Model file for the job. Use its own axes, mm. Face numbers are marked on the shaded views. A direction names the side the tool comes from. Round coordinates to 2 decimals unless told otherwise and drop trailing zeros. Loops run counter-clockwise (first coordinate to the right, second up) from the corner with the lowest first, then second, coordinate; pieces in that order, holes last. Notation, with made-up numbers: (75.5, 5) - (122.5, 5) arc R23 cw to (122.5, 13) - close; hole circle Ø7 at (71, 84). An arc over 180 degrees is marked (long way). Answer as a JSON object with one key per item and string values.
from build123d import *

# Parameters (mm, degrees)
F2_W = 40.0049984455
F2_H = 8.5304779932


with BuildPart() as f1:
    # F0 (on Front) → F1 (revolve)
    with BuildSketch(Plane.XZ):
        with BuildLine():
            Line((-17.918098104, 0), (0, 0))
            Line((0, 0), (0, 10.5895595625))
            Line((0, 10.5895595625), (-17.918098104, 10.5895595625))
            ThreePointArc((-17.918098104, 10.5895595625), (-36.5355256935, 5.2947797813), (-17.918098104, 0))
        make_face()
    revolve(axis=Axis((0, 0, 5.2947797813), (0, 0, 1)))

    # F2 (on Front) → F3 (revolve)
    with BuildSketch(Plane.XZ):
        with Locations((-20.0024992228, 4.2652389966)):
            Rectangle(F2_W, F2_H)
        with BuildLine():
            ThreePointArc((-40.0049984455, 8.5304779932), (-44.2702374421, 4.2652389966), (-40.0049984455, 0))
            Line((-40.0049984455, 0), (-40.0049984455, 8.5304779932))
        make_face()
    revolve(axis=Axis((0, 0, 4.2652389966), (0, 0, 1)))

    # F4 (on Front) → F5 (revolve)
    with BuildSketch(Plane.XZ):
        Polygon((-47.0647066832, 0), (0, 0), (0, 5.5889338255), (-46.6507802162, 5.5889338255), (-45.9072005883, 1.7057990241), align=None)
        Polygon((-48.222212778, -1.7057990241), (-47.0647066832, 0), (-51.1828698218, 0), (-51.1828698218, 5.5889338255), (-46.6507802162, 5.5889338255), (-46.682603885, 5.7551239565), (-50.0942019331, 8.0701361462), (-54.1435268656, 7.2947328496), (-56.4585390553, 3.8831348014), (-55.6831357586, -0.166190131), (-52.2715377104, -2.4812023207), align=None)
        Polygon((-51.1828698218, 0), (-47.0647066832, 0), (-45.9072005883, 1.7057990241), (-46.6507802162, 5.5889338255), (-51.1828698218, 5.5889338255), align=None)
    revolve(axis=Axis((0, 0, 2.7944669127), (0, 0, 1)))


solid = f1.part
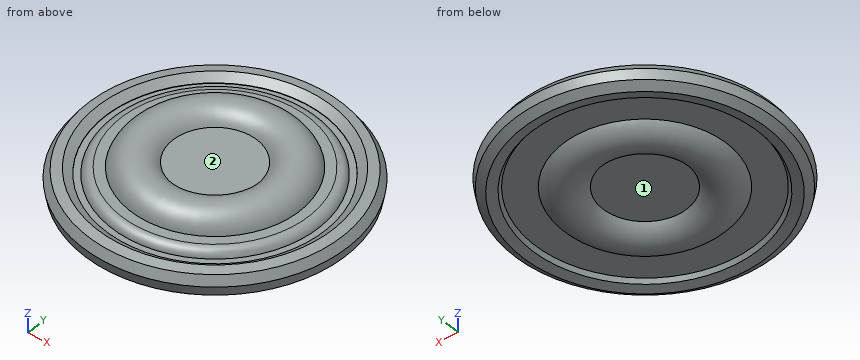
1) Tool access for the marked faces 1 and 2: list every direction of +Z, -Z, +X, -X, +Y, -Y with a clear straight run to the whole face (end or side of a thin tool).
Values follow:
{"face 1": "-Z", "face 2": "+Z"}
2) Drop flat-ended pins along their axis: P1, Ø6, axis at x = -40.5, z = 8, coming from the -Y side; P2, Ø11, axis at x = -6.5, y = -7.5, coming from the -Z side; P3, Ø4, axis at y = 18, z = -1, coming from the +X side; P4, Ø5, axis at x = -26.5, y = 3, coming from the -Z side. Give the stop position or say it passes through.
Values follow:
{"P1": "y = -39.54", "P2": "z = 0", "P3": "x = 53.29", "P4": "z = -4.77"}
3) Slice it at C-C on z = 12.25. List the corners of the cut face in (x, y).
Values follow:
{"outline": "circle Ø67.49 at (0, 0); hole circle Ø38.41 at (0, 0)"}
4) Probe probe 1 along X at (y, z) = (-12, 6.5); probe 2 along X at (y, z) = (-24, -1.5); probe 3 along Z at (x, y) = (-33.5, -16). List the from-to ranges inside material, lowest first.
Values follow:
{"probe 1": "-53.35 to -46.25, -41.96 to 41.96, 46.25 to 53.35", "probe 2": "-48.06 to -41.66, -23.93 to 23.93, 41.66 to 48.06", "probe 3": "0 to 8.53"}
